Build history of the part. All positions in model axes, mm. Face numbers are marked on the shaded views. A direction names the side the tool comes from. Give positions to 0.01 mm unless a question says otherwise; leave off trailing zeros. Loops run counter-clockwise (first coordinate to the right, second up) from the corner with the lowest first, then second, coordinate; pieces in that order, holes last. Notation, with made-up numbers: M 72,-23.5 L 86,-23.5 A15 ccw 86,-6.5 Z; hole C 39,-34.75 d1. An arc over 180 degrees is marked long. Answer as a JSON object with one key per item and string values. Group by question number.
1. Slice it at D-D (z = 3.5). List the corners of the cut face in (x, y), then the cut area to 3 significant figures.
2. Drop flat-ended pins along their axis: pin 1 Ø1 at (y, z) = (13.85, 7.1) entering from +X; pin 2 Ø12 at (y, z) = (-5, 10) entering from -X; pin 3 Ø1.5 at (y, z) = (-5.5, 5.5) entering from -X; pin 4 Ø13 at (x, y) = (-2, 2.5) entering from +Z. Give the stop position or say it passes through.
3. Slice it at A-A (y = -1). Give the number of separate pieces and of enclosed holes in the cut face, then the cut area to 3 significant figures.
4. Mould opens along X. For the marked faces 1, 2 and 3 say: released by +X, released by -X, zero draft, split by the parting line, or undercut.
5. Slice it at C-C (y = -13.85). List the corners of the cut face in (x, z), then the cut area to 3 significant figures.
6. Drill centre lines: line 1 along Y through (x, z) = (11.75, 7.1); line 2 along Y through (x, z) = (9.25, 7.1); line 3 along Z through (x, y) = (10.5, 5.25). Where is each one in solid material? Low to high. Write a range as [from, to].
7. Slice it at B-B (z = 7). List the corners of the cut face in (x, y), then the cut area to 3 significant figures.
8. 3-axis set-ups, long thin cutter, end or side, ignore diameter. For the marked faces 4, 5 and 6: which of +Z, -Z, +X, -X, +Y, -Y reach the whole face in a straight line?
from build123d import *

# Parameters (mm, degrees)
SKETCH1_R                = 3.75
BOSS_EXTRUDE1_DEPTH      = 5
CUT_EXTRUDE2_DEPTH       = 2
BOSS_EXTRUDE2_DEPTH      = 3.5
BOSS_EXTRUDE2_DEPTH_BACK = 4
SKETCH5_R                = 0.8
SKETCH6_W                = 12.2
SKETCH6_H                = 23.2
CUT_EXTRUDE3_DEPTH       = 4


with BuildPart() as part:
    # Sketch1 → Boss-Extrude1 (new body)
    with BuildSketch(Plane.XY):
        with BuildLine():
            Line((10, -17.5), (-5, -17.5))
            ThreePointArc((-5, -17.5), (-8.535533906, -16.035533906), (-10, -12.5))
            Line((-10, -12.5), (-10, 12.5))
            ThreePointArc((-10, 12.5), (-8.535533906, 16.035533906), (-5, 17.5))
            Line((-5, 17.5), (10, 17.5))
            Line((10, 17.5), (10, -17.5))
        make_face()
        Circle(SKETCH1_R, mode=Mode.SUBTRACT)
    extrude(amount=-BOSS_EXTRUDE1_DEPTH)

    # Sketch3 → Cut-Extrude2 (cut)
    with BuildSketch(Plane.XY):
        with BuildLine():
            Line((-1.984313483, 14.25), (-3.720587781, 0.46875))
            ThreePointArc((-3.720587781, 0.46875), (-3.75, 0), (-3.720587781, -0.46875))
            Line((-3.720587781, -0.46875), (-1.984313483, -14.25))
            ThreePointArc((-1.984313483, -14.25), (0, -16), (1.984313483, -14.25))
            Line((1.984313483, -14.25), (3.720587781, -0.46875))
            ThreePointArc((3.720587781, -0.46875), (3.75, 0), (3.720587781, 0.46875))
            Line((3.720587781, 0.46875), (1.984313483, 14.25))
            ThreePointArc((1.984313483, 14.25), (0, 16), (-1.984313483, 14.25))
        make_face()
    extrude(amount=-CUT_EXTRUDE2_DEPTH, mode=Mode.SUBTRACT)

    # Sketch5 → Boss-Extrude2 (add, two sides: drawn at the far end of the back side and taken through both)
    with BuildSketch(Plane(origin=(10, 0, 0), x_dir=(0, 0, -1), z_dir=(1, 0, 0)).offset(-BOSS_EXTRUDE2_DEPTH_BACK)):
        with BuildLine():
            Line((5, 17.5), (-10.2, 17.5))
            ThreePointArc((-10.2, 17.5), (-13.735533906, 16.035533906), (-15.2, 12.5))
            Line((-15.2, 12.5), (-15.2, -12.5))
            ThreePointArc((-15.2, -12.5), (-13.735533906, -16.035533906), (-10.2, -17.5))
            Line((-10.2, -17.5), (5, -17.5))
            Line((5, -17.5), (5, 17.5))
        make_face()
        with Locations((-7.1, 13.85)):
            Circle(SKETCH5_R, mode=Mode.SUBTRACT)
        with Locations((-7.1, -13.85)):
            Circle(SKETCH5_R, mode=Mode.SUBTRACT)
        with BuildLine():
            ThreePointArc((-4.006634299, -0.1808), (-7.1, 11.5), (-10.193365701, -0.1808))
            ThreePointArc((-10.193365701, -0.1808), (-7.1, -4.2), (-4.006634299, -0.1808))
        make_face(mode=Mode.SUBTRACT)
    extrude(amount=BOSS_EXTRUDE2_DEPTH + BOSS_EXTRUDE2_DEPTH_BACK)

    # Sketch6 → Cut-Extrude3 (cut)
    with BuildSketch(Plane.ZY.offset(-6)):
        with Locations((7.1, 0)):
            Rectangle(SKETCH6_W, SKETCH6_H)
    extrude(amount=-CUT_EXTRUDE3_DEPTH, mode=Mode.SUBTRACT)


solid = part.part
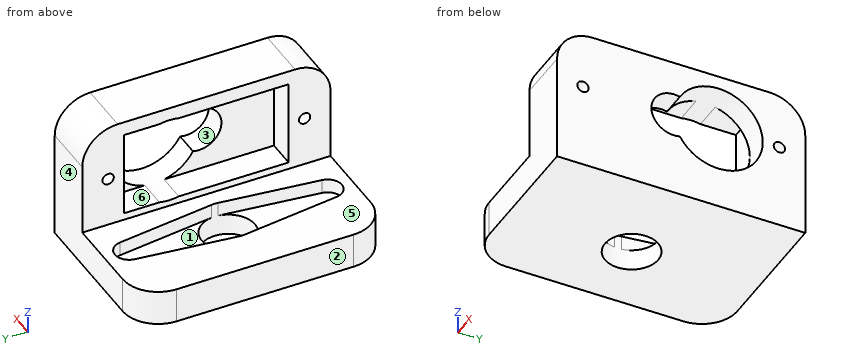
Established:
{
 "1": {"outline": "M 6,-17.5 L 13.5,-17.5 L 13.5,0.14 L 10,0.14 L 10,-11.6 L 6,-11.6 Z; M 6,11.6 L 10,11.6 L 10,10.36 L 13.5,10.36 L 13.5,17.5 L 6,17.5 Z", "area": "134 mm^2"},
 "2": {"pin 1": "passes through", "pin 2": "stops at x = 6", "pin 3": "stops at x = 10", "pin 4": "stops at z = 0"},
 "3": {"separate pieces": "3", "enclosed holes": "0", "area": "124 mm^2"},
 "4": {"face 1": "undercut", "face 2": "released by -X", "face 3": "zero draft"},
 "5": {"outline": "M -9.81,-5 L 13.5,-5 L 13.5,6.3 L 6,6.3 L 6,0 L 2.03,0 L 2.03,-2 L -2.03,-2 L -2.03,0 L -9.81,0 Z; M 6,7.9 L 13.5,7.9 L 13.5,15.01 L 6,15.01 Z", "area": "209 mm^2"},
 "6": {"line 1": "y = [-17.5, -14.65], [-13.05, -4.2], [11.5, 13.05], [14.65, 17.5]", "line 2": "y = [-17.5, -14.65], [-13.05, -11.6], [11.6, 13.05], [14.65, 17.5]", "line 3": "z = [-5, 0.85], [13.35, 15.2]"},
 "7": {"outline": "M 6,-17.5 L 13.5,-17.5 L 13.5,-14.64 L 6,-14.64 Z; M 6,-13.06 L 13.5,-13.06 L 13.5,-4.2 L 10,-4.2 L 10,-11.6 L 6,-11.6 Z; M 6,11.6 L 10,11.6 L 10,11.5 L 13.5,11.5 L 13.5,13.06 L 6,13.06 Z; M 6,14.64 L 13.5,14.64 L 13.5,17.5 L 6,17.5 Z", "area": "90.9 mm^2"},
 "8": {"face 4": "+Z, -Z, +X, -X, +Y", "face 5": "+Z, -X, +Y, -Y", "face 6": "-X"}
}
